Model file for the job. Use its own axes, mm. Coordinates: 2 decimals unless noted, no trailing zeros. Return JSON: item names as keys, results as strings.
```python
from build123d import *

# Parameters (mm, degrees)
SKETCH1_W                        = 249.301
SKETCH1_H                        = 787.4
BOSS_EXTRUDE1_DEPTH              = 6.35
F_10_CLEARANCE_HOLE1_D           = 5.6134
F_10_CLEARANCE_HOLE1_CSINK_D     = 6.8834
F_10_CLEARANCE_HOLE1_CSINK_ANGLE = 90
CUT_EXTRUDE1_DEPTH               = 840.858019251


with BuildPart() as part:
    # Sketch1 → Boss-Extrude1 (new body)
    with BuildSketch(Plane.XY):
        with Locations((167.4495, 393.7)):
            Rectangle(SKETCH1_W, SKETCH1_H)
    extrude(amount=BOSS_EXTRUDE1_DEPTH)

    # #10 Clearance Hole1 (through all)
    with Locations(Plane.XY.offset(6.35)):
        with Locations((49.149, 552.45), (49.149, 527.05), (49.149, 260.35), (49.149, 234.95)):
            CounterSinkHole(F_10_CLEARANCE_HOLE1_D / 2, F_10_CLEARANCE_HOLE1_CSINK_D / 2, counter_sink_angle=F_10_CLEARANCE_HOLE1_CSINK_ANGLE)

    # Sketch6 → Cut-Extrude1 (cut, through all)
    with BuildSketch(Plane.XY.offset(6.35)):
        with BuildLine():
            Line((292.1, 495.3), (304.8, 495.3))
            Line((304.8, 495.3), (304.8, 292.1))
            Line((304.8, 292.1), (292.1, 292.1))
            ThreePointArc((292.1, 292.1), (288.807245657, 309.197898263), (279.4, 323.85))
            ThreePointArc((279.4, 323.85), (269.992754343, 338.502101737), (266.7, 355.6))
            Line((266.7, 355.6), (266.7, 431.8))
            ThreePointArc((266.7, 431.8), (269.992754343, 448.897898263), (279.4, 463.55))
            ThreePointArc((279.4, 463.55), (288.807245657, 478.202101737), (292.1, 495.3))
        make_face()
    extrude(amount=-CUT_EXTRUDE1_DEPTH, mode=Mode.SUBTRACT)


solid = part.part
```
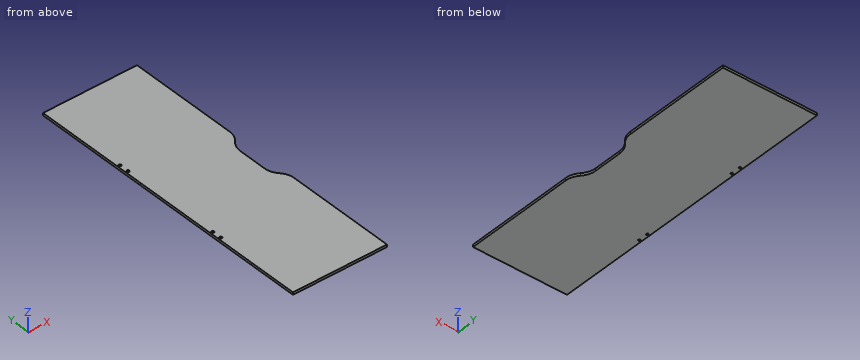
Item 1: Drop a flat-ended pin along its axis: pin 1 Ø1.9 at (y, z) = (406, 4) entering from +X. Give the stop position or say it passes through.
Check result:
{"pin 1": "stops at x = 266.7"}
Item 2: Saw through at A-A (z = 4). Count the separate pieces of the cut face and the enclosed holes in it, and give its area (3 significant figures).
Check result:
{"separate pieces": "1", "enclosed holes": "4", "area": "193,000 mm2"}
Item 3: Wall check: line 1 (X direction, y = 234.95, z = 2.55); line 2 (X direction, y = 294, z = 2); line 3 (X direction, y = 392, z = 3.5). Give the ranges that are in metal, low to high.
Check result:
{"line 1": "x = 42.8 to 46.34, 51.96 to 292.1", "line 2": "x = 42.8 to 292.06", "line 3": "x = 42.8 to 266.7"}
